Verification items for the finished model (mm, model axes). A direction names the side the tool comes from. Round coordinates to 2 decimals unless told otherwise and drop trailing zeros. Write each loop counter-clockwise with the first axis right and the second up, starting at its lowest first coordinate (ties: lowest second). Pieces come first, ordered by that corner, then holes. Notation, with made-up numbers: (0, 58.5) - (25, 58.5) arc R12 ccw to (25, 68.5) - close; hole circle Ø10 at (-10.75, -8.75). An arc over 180 degrees is marked (long way). Answer as a JSON object with one key per item and string values.
```python
from build123d import *

# Parameters (mm, degrees)
F1_DEPTH = 5.953125


with BuildPart() as f1:
    # F0 (on Right) → F1 (new body)
    with BuildSketch(Plane.YZ):
        Polygon((-69.85, 72.489666), (-76.2, 72.489666), (-76.2, 47.089666), (-70.246875, 47.089666), (-70.246875, 8.989666), (-76.2, 8.989666), (-76.2, -9.663459), (-70.246875, -9.663459), (-70.246875, -47.763459), (-76.2, -47.763459), (-76.2, -79.910334), (76.2, -79.910334), (76.2, -54.510334), (69.85, -54.510334), (69.85, -60.463459), (57.15, -60.463459), (57.15, -54.510334), (50.8, -54.510334), (50.8, -29.110334), (44.45, -29.110334), (44.45, -35.063459), (31.75, -35.063459), (31.75, -29.110334), (25.4, -29.110334), (25.4, -3.710334), (19.05, -3.710334), (19.05, -9.663459), (6.35, -9.663459), (6.35, -3.710334), (0, -3.710334), (0, 21.689666), (-6.35, 21.689666), (-6.35, 15.736541), (-19.05, 15.736541), (-19.05, 21.689666), (-25.4, 21.689666), (-25.4, 47.089666), (-31.75, 47.089666), (-31.75, 41.136541), (-44.45, 41.136541), (-44.45, 47.089666), (-50.8, 47.089666), (-50.8, 72.489666), (-57.15, 72.489666), (-57.15, 66.536541), (-69.85, 66.536541), align=None)
    extrude(amount=F1_DEPTH)


solid = f1.part
```
Q1. Section check B-B, the plane z = 4. Record the cut outline in (x, y).
Geometry check:
{"outline": "(0, -76.2) - (5.95, -76.2) - (5.95, 0) - (0, 0) - close"}
Q2. Release check for a two-part mould opening along Y. For faces 1 (the flat face through (3, -73, 8.99)), 2 (the flat face through (3, -69.85, 69)), 3 (the flat face through (3, 25.4, -17)), 4 (the flat face through (3, 64, -60.463)) record: released by +Y, released by -Y, zero draft, split by the parting line, or undercut.
Geometry check:
{"face 1": "zero draft", "face 2": "undercut", "face 3": "released by +Y", "face 4": "undercut"}
Q3. Material ranges on line 1 along Y through (x, z) = (4.95, 45); line 2 along Y through (x, z) = (3.6, 18); line 3 along Y through (x, z) = (5.6, 8.5), recorded low to high. Write a range as [from, to].
Geometry check:
{"line 1": "y = [-70.25, -44.45], [-31.75, -25.4]", "line 2": "y = [-70.25, -19.05], [-6.35, 0]", "line 3": "y = [-76.2, 0]"}
Q4. Section check A-A, the plane y = -36. Record the cut outline in (x, z).
Geometry check:
{"outline": "(0, -79.91) - (5.95, -79.91) - (5.95, 41.14) - (0, 41.14) - close"}
Q5. Gauge pin test, flat ends, axial feed: P1, Ø1.8, axis at x = 1.5, y = -38, coming from the +Z side; P2, Ø3, axis at x = 3.5, z = 58.5, coming from the +Y side; P3, Ø2, axis at x = 1, z = 11.5, coming from the -Y side. Record the tip position at first contact, or that the pin passes through.
Geometry check:
{"P1": "stops at z = 41.14", "P2": "stops at y = -50.8", "P3": "stops at y = -70.25"}
Q6. Set-up check for faces 5 (the flat face through (3, -73, -9.663)), 6 (the flat face through (3, 73, -54.51)), 7 (the flat face through (3, -38, 41.137)), 8 (the flat face through (3, -1, -79.91)): record each of +Z, -Z, +X, -X, +Y, -Y from which the full face is reachable in a straight line by a thin tool's end or side.
Geometry check:
{"face 5": "+X, -X, -Y", "face 6": "+Z, +X, -X, +Y", "face 7": "+Z, +X, -X", "face 8": "-Z, +X, -X, +Y, -Y"}
